Geometry check sheet. Reference: the model listing, model coordinates, mm. Face numbers are marked on the shaded views. A direction names the side the tool comes from. Give positions to 0.01 mm unless a question says otherwise; leave off trailing zeros. Loops run counter-clockwise (first coordinate to the right, second up) from the corner with the lowest first, then second, coordinate; pieces in that order, holes last. Notation, with made-up numbers: (-26.5, 85) -> (5.5, 85) arc R16 cw to (5.5, 103) -> close; hole circle Ø11 at (29.5, 31.5). An arc over 180 degrees is marked (long way). Answer as a JSON object with one key per item and string values.
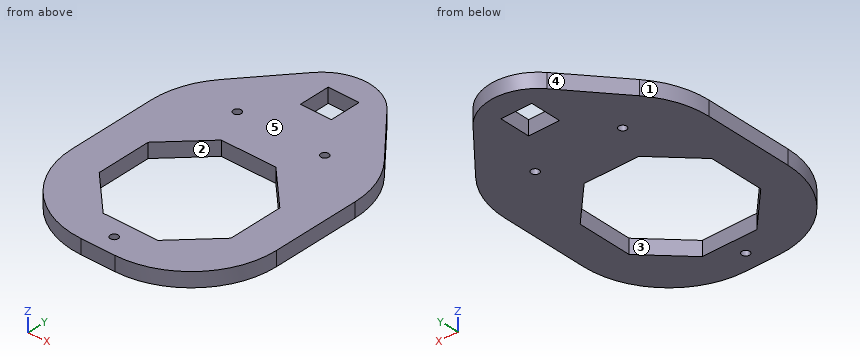
from build123d import *

# Parameters (mm, degrees)
F0_R     = 1.6
F0_W     = 12.72
F0_H     = 12.72
F1_DEPTH = 6
F2_R     = 35
F3_R     = 20


with BuildPart() as f1:
    # F0 (on Top) → F1 (new body)
    with BuildSketch(Plane.XY):
        Polygon((27.1, 118.708467), (-14.9, 69.1), (-14.9, -14.9), (69.1, -14.9), (69.1, 69.1), align=None)
        with Locations((27.1, -7.45)):
            Circle(F0_R, mode=Mode.SUBTRACT)
        Polygon((0, 15.874812), (0, 38.325188), (15.874812, 54.2), (38.325188, 54.2), (54.2, 38.325188), (54.2, 15.874812), (38.325188, 0), (15.874812, 0), align=None, mode=Mode.SUBTRACT)
        with Locations((9.1, 69.1)):
            Circle(F0_R, mode=Mode.SUBTRACT)
        with Locations((45.1, 69.1)):
            Circle(F0_R, mode=Mode.SUBTRACT)
        with Locations((27.1, 91.46)):
            Rectangle(F0_W, F0_H, mode=Mode.SUBTRACT)
    extrude(amount=F1_DEPTH)

    # F2
    f2_edges = [f1.edges().sort_by_distance(p)[0] for p in [
        (69.1, -14.9, 3),
        (-14.9, -14.9, 3),
        (-14.9, 69.1, 3),
        (69.1, 69.1, 3),
    ]]
    fillet(f2_edges, radius=F2_R)

    # F3
    f3_edges = [f1.edges().sort_by_distance(p)[0] for p in [
        (27.1, 118.708467, 3),
    ]]
    fillet(f3_edges, radius=F3_R)


solid = f1.part
1) Section check C-C on y = 9.5. Record the cut outline in (x, z), plus the area to 3 significant figures.
Geometry check:
{"outline": "(-13.26, 0) -> (6.37, 0) -> (6.37, 6) -> (-13.26, 6) -> close; (47.83, 0) -> (67.46, 0) -> (67.46, 6) -> (47.83, 6) -> close", "area": "236 mm2"}
2) Material ranges on line 1 along Y through (x, z) = (45.1, 2.6); line 2 along Y through (x, z) = (27.1, 2.95); line 3 along X through (y, z) = (69.1, 2.5), recorded low to high. Write a range as from..to.
Geometry check:
{"line 1": "y = -13.13..6.77, 47.43..67.5, 70.7..97.45", "line 2": "y = -14.9..-9.05, -5.85..0, 54.2..85.1, 97.82..107.76", "line 3": "x = -12.47..7.5, 10.7..43.5, 46.7..66.67"}
3) Depth check by flat-ended pin: P1, Ø5, axis at x = 50.5, y = 78, coming from the -Z side; P2, Ø1.8, axis at y = 88.5, z = 2, coming from the -X side; P3, Ø3, axis at y = 93.5, z = 2, coming from the +X side; P4, Ø1.8, axis at x = 25, z = 4, coming from the +Y side. Enter the tip coordinate at first touch or a pass-through.
Geometry check:
{"P1": "stops at z = 0", "P2": "stops at x = 0.76", "P3": "stops at x = 49.71", "P4": "stops at y = 107.72"}
4) Section check D-D on y = 69.1. Record the cut outline in (x, z), plus the area to 3 significant figures.
Geometry check:
{"outline": "(-12.47, 0) -> (7.5, 0) -> (7.5, 6) -> (-12.47, 6) -> close; (10.7, 0) -> (43.5, 0) -> (43.5, 6) -> (10.7, 6) -> close; (46.7, 0) -> (66.67, 0) -> (66.67, 6) -> (46.7, 6) -> close", "area": "436 mm2"}
5) Draft check along Y on the marked faces 3, 4 and 5. Enter one of: pulls with the +Y half, pulls with the -Y half, needs draft (parallel to the pull), parting line crosses it, or undercut.
Geometry check:
{"face 3": "undercut", "face 4": "pulls with the +Y half", "face 5": "needs draft"}
6) Section check A-A on x = 27.1. Record the cut outline in (y, z), plus the area to 3 significant figures.
Geometry check:
{"outline": "(-14.9, 0) -> (-9.05, 0) -> (-9.05, 6) -> (-14.9, 6) -> close; (-5.85, 0) -> (0, 0) -> (0, 6) -> (-5.85, 6) -> close; (54.2, 0) -> (85.1, 0) -> (85.1, 6) -> (54.2, 6) -> close; (97.82, 0) -> (107.76, 0) -> (107.76, 6) -> (97.82, 6) -> close", "area": "315 mm2"}
7) Section check B-B on z = 3.35. Record the cut outline in (x, y), plus the area to 3 significant figures.
Geometry check:
{"outline": "(-14.9, 20.1) arc R35 ccw to (20.1, -14.9) -> (34.1, -14.9) arc R35 ccw to (69.1, 20.1) -> (69.1, 56.27) arc R35 ccw to (60.81, 78.89) -> (42.36, 100.68) arc R20 ccw to (11.84, 100.68) -> (-6.61, 78.89) arc R35 ccw to (-14.9, 56.27) -> close; hole (0, 15.87) -> (15.87, 0) -> (38.33, 0) -> (54.2, 15.87) -> (54.2, 38.33) -> (38.33, 54.2) -> (15.87, 54.2) -> (0, 38.33) -> close; hole circle Ø3.2 at (9.1, 69.1); hole (20.74, 85.1) -> (33.46, 85.1) -> (33.46, 97.82) -> (20.74, 97.82) -> close; hole circle Ø3.2 at (27.1, -7.45); hole circle Ø3.2 at (45.1, 69.1)", "area": "5,830 mm2"}
8) Tool access check on the marked faces 1 and 2. Record the directions out of +Z, -Z, +X, -X, +Y, -Y that give a thin tool (end or side, any length) a straight path to the whole face; none if there is none.
Geometry check:
{"face 1": "+Z, -Z, -X, +Y", "face 2": "+Z, -Z"}
